For this review, take the finished solid that the model builds, in its own axes (mm). A direction names the side the tool comes from. Round coordinates to 2 decimals unless told otherwise and drop trailing zeros. Order: outer loops, then holes, each group sorted by start corner. A loop starts at its lowest first (then second) coordinate and runs counter-clockwise, first axis right, second up. Notation, with made-up numbers: M -21.5,30 L -8.5,30 A34 cw -8.5,64 Z; hole C 87,32 d9. An arc over 180 degrees is marked long. Use a Markdown table: item, result.
from build123d import *

# Parameters (mm, degrees)
SKETCH5_R           = 3.175
BOSS_EXTRUDE3_DEPTH = 101.6
BOSS_EXTRUDE4_DEPTH = 3.96875
SKETCH8_OUTSIDE_W   = 404.842
SKETCH8_OUTSIDE_H   = 406.562
SKETCH8_OUTSIDE_R   = 5.55625
CUT_EXTRUDE3_DEPTH  = 106.909373724
CUT_EXTRUDE3_DRAFT  = -60
CUT_EXTRUDE4_DEPTH  = 0.254
CIRPATTERN1_COUNT   = 3


with BuildPart() as part:
    # Sketch5 → Boss-Extrude3 (new body)
    with BuildSketch(Plane(origin=(52.784375, 0, 0), x_dir=(0, 0, -1), z_dir=(1, 0, 0))):
        Circle(SKETCH5_R)
    extrude(amount=-BOSS_EXTRUDE3_DEPTH)

    # Sketch11 → Revolve1 (revolve)
    with BuildSketch(Plane.XY):
        Polygon((-48.815625, 3.175), (-48.815625, 0), (36.909375, 0), (33.734375, 3.175), align=None)
    revolve(axis=Axis((-48.815625, 0, 0), (1, 0, 0)))

    # Sketch6 → Boss-Extrude4 (add)
    with BuildSketch(Plane.ZY.offset(48.815625)):
        Polygon((5.55625, 3.207902433), (0, 6.415804866), (-5.55625, 3.207902433), (-5.55625, -3.207902433), (0, -6.415804866), (5.55625, -3.207902433), align=None)
    extrude(amount=BOSS_EXTRUDE4_DEPTH)


with BuildPart() as cut_extrude3_tool:
    # Sketch8 outside → Cut-Extrude3 (with draft: the straight prism first)
    with BuildSketch(Plane.ZY.offset(52.784375)):
        Rectangle(SKETCH8_OUTSIDE_W, SKETCH8_OUTSIDE_H)
        Circle(SKETCH8_OUTSIDE_R, mode=Mode.SUBTRACT)
    extrude(amount=-CUT_EXTRUDE3_DEPTH)
    # Cut-Extrude3: the draft: its side faces are tilted about the plane it starts from
    cut_extrude3_sides = [cut_extrude3_tool.faces().sort_by_distance(p)[0] for p in [
        (0.670311862, -203.281, 0),
        (0.670311862, 0, 202.421),
        (0.670311862, 203.281, 0),
        (0.670311862, 0, -202.421),
        (0.670311862, 0, -5.55625),
    ]]
    draft(cut_extrude3_sides, Plane.ZY.offset(52.784375), CUT_EXTRUDE3_DRAFT)


with BuildPart() as part_1:
    add(part.part)

    # Cut-Extrude3: cut by cut_extrude3_tool
    add(cut_extrude3_tool.part, mode=Mode.SUBTRACT)

    # Sketch12 → Cut-Extrude4 (cut)
    with BuildSketch(Plane.ZY.offset(52.784375)):
        with BuildLine():
            Line((0.1666875, 4.2783125), (0.1666875, 2.3891875))
            ThreePointArc((0.1666875, 2.3891875), (0, 2.2225), (-0.1666875, 2.3891875))
            Line((-0.1666875, 2.3891875), (-0.1666875, 4.2783125))
            ThreePointArc((-0.1666875, 4.2783125), (0, 4.445), (0.1666875, 4.2783125))
        make_face()
    cut_extrude4 = extrude(amount=-CUT_EXTRUDE4_DEPTH, mode=Mode.SUBTRACT)

    # CirPattern1: Cut-Extrude4 ×3 about axis
    cirpattern1_axis = Axis((0, 0, 0), (1, 0, 0))
    for i in range(1, CIRPATTERN1_COUNT):
        add(cut_extrude4.rotate(cirpattern1_axis, i * 360 / CIRPATTERN1_COUNT), mode=Mode.SUBTRACT)


solid = part_1.part
Q1. Add section A-A (x = -43). Write out the cut boundary in (y, z) (3 decimals).
Determined:
| item | result |
|---|---|
| outline | C 0,0 d6.35 |
Q2. Clearance check with flat-ended pins moving along their axes: pin 1 (1.5 mm diameter, centred on x = 39.5, y = -0.5, fed in from +Z) (3 decimals); pin 2 (4 mm diameter, centred on x = -3.5, z = -1.5, fed in from +Y) (3 decimals); pin 3 (1 mm diameter, centred on x = 7.5, y = 1, fed in from +Z). State where each tip first meets the part, or that it passes through.
Determined:
| item | result |
|---|---|
| pin 1 | stops at z = 3.175 |
| pin 2 | stops at y = 3.175 |
| pin 3 | stops at z = 3.14 |
Q3. Wall thickness on line 1 along X through (y, z) = (-3.5, 4); line 2 along Y through (x, z) = (-14, 1.5); line 3 along Y through (x, z) = (45, 2.5): over which ranges is each line inside the solid? List them lowest first. Write a range as [from, to].
Determined:
| item | result |
|---|---|
| line 1 | x = [-52.78, -48.82] |
| line 2 | y = [-2.8, 2.8] |
| line 3 | y = [-1.96, 1.96] |
Q4. Machinability: for faces 1 (the flat face through (-48.816, -3, -3)), 2 (the conical face through (-52.67, -2.89, 4.98)), which of the approach directions +Z, -Z, +X, -X, +Y, -Y give a long, thin tool a straight path to every point of the face, cutting with its end or side? Answer none if there is none.
Determined:
| item | result |
|---|---|
| face 1 | +X |
| face 2 | +Z, -X, -Y |
